Autodesk Fusion 360 part; units mm, degrees
sketch "Skizze1" plane through (0, 0, 0) normal (0, 1, 0) x (1, 0, 0)
  circle A0 centre (0, 0) radius 4
  dimension "d1" = 8
extrude "Extrusion1" add sketch "Skizze1" along normal blind 300
fillet "Abrundung1" radius 4 1 edges at (-3.7293, 0, 1.4465)
fillet "Abrundung2" radius 4 1 edges at (-3.7293, 300, 1.4465)
The listing builds one solid part. Answer for the finished solid, in the listing's coordinates (mm). Give positions to 0.01 mm unless a question says otherwise; leave off trailing zeros. Order: outer loops, then holes, each group sorted by start corner. A loop starts at its lowest first (then second) coordinate and runs counter-clockwise, first axis right, second up. Notation, with made-up numbers: M -10.75,-13 L 38.25,-13 A23 ccw 38.25,17 Z; hole C -24.5,-5.75 d7. An arc over 180 degrees is marked long. Put each result on its own line as item: value. Start each with the question number.
Item 1: Flat-ended cylindrical pins translate along their axes: P1, Ø1.5, axis at x = 1, z = 3, coming from the -Y side; P2, Ø2, axis at x = -1.5, z = -0.5, coming from the +Y side; P3, Ø3, axis at y = 167.5, z = 3, coming from the -X side. Find the tip coordinate at first contact, or state that the pin passes through.
Item 2: Find the intervals of material crossed by line 1 along Z through (x, y) = (-0.5, 50); line 2 along Y through (x, z) = (0, 1.25), in increasing order.
Item 3: The part is cut by section C-C, the plane x = -2. Determine the outline of the cut face in (y, z).
Item 4: The part is cut by section B-B, the plane z = -2.75. Determine the outline of the cut face in (x, y), and give its area (3 significant figures).
Item 5: The part is cut by section A-A, the plane y = 95.5. Determine the outline of the cut face in (x, z).
Answer key:
1. P1: stops at y = 0.81
1. P2: stops at y = 299.96
1. P3: stops at x = -3.71
2. line 1: z = -3.97 to 3.97
2. line 2: y = 0.2 to 299.8
3. outline: M 4,-3.46 L 296,-3.46 A3.46 ccw 296,3.46 L 4,3.46 A3.46 ccw Z
4. outline: M -2.9,4 A2.9 ccw 2.9,4 L 2.9,296 A2.9 ccw -2.9,296 Z
4. area: 1,720 mm²
5. outline: C 0,0 d8
